from build123d import *

# Parameters (mm, degrees)
ESQUISSE1_R               = 7
ESQUISSE1_R_2             = 6
BOSS_EXTRU_1_DEPTH        = 2.5
BOSS_EXTRU_1_DEPTH_BACK   = 2.5
ESQUISSE1_R_3             = 10.5
ESQUISSE1_R_4             = 9.5
BOSS_EXTRU_1_2_DEPTH      = 2.5
BOSS_EXTRU_1_2_DEPTH_BACK = 2.5
ESQUISSE1_3_R             = 9.5
ESQUISSE1_3_R_2           = 7
BOSS_EXTRU_2_DEPTH        = 2
BOSS_EXTRU_2_DEPTH_BACK   = 2


with BuildPart() as part:
    # Esquisse1 → Boss.-Extru.1 (new body, two sides)
    with BuildSketch(Plane(origin=(0, 0, 0), x_dir=(1, 0, 0), z_dir=(0, 1, 0))) as boss_extru_1_sk:
        Circle(ESQUISSE1_R)
        Circle(ESQUISSE1_R_2, mode=Mode.SUBTRACT)
    extrude(amount=BOSS_EXTRU_1_DEPTH)
    extrude(boss_extru_1_sk.sketch, amount=-BOSS_EXTRU_1_DEPTH_BACK)



with BuildPart() as body_2:
    # Esquisse1 → Boss.-Extru.1 2 (new body, two sides)
    with BuildSketch(Plane(origin=(0, 0, 0), x_dir=(1, 0, 0), z_dir=(0, 1, 0))) as boss_extru_1_2_sk:
        Circle(ESQUISSE1_R_3)
        Circle(ESQUISSE1_R_4, mode=Mode.SUBTRACT)
    extrude(amount=BOSS_EXTRU_1_2_DEPTH)
    extrude(boss_extru_1_2_sk.sketch, amount=-BOSS_EXTRU_1_2_DEPTH_BACK)


with BuildPart() as part_1:
    add(part.part)

    add(body_2.part)  # Boss.-Extru.2 merges body 2
    # Esquisse1_3 → Boss.-Extru.2 (add, two sides)
    with BuildSketch(Plane(origin=(0, 0, 0), x_dir=(1, 0, 0), z_dir=(0, 1, 0))) as boss_extru_2_sk:
        Circle(ESQUISSE1_3_R)
        Circle(ESQUISSE1_3_R_2, mode=Mode.SUBTRACT)
    extrude(amount=BOSS_EXTRU_2_DEPTH)
    extrude(boss_extru_2_sk.sketch, amount=-BOSS_EXTRU_2_DEPTH_BACK)


solid = part_1.part
Part model, mm, in its own coordinate system. A direction names the side the tool comes from. Coordinates: 2 decimals unless noted, no trailing zeros. Order: outer loops, then holes, each group sorted by start corner. A loop starts at its lowest first (then second) coordinate and runs counter-clockwise, first axis right, second up. Notation, with made-up numbers: (18.25, 57) - (31.25, 57) arc R11 cw to (31.25, 75) - close; hole circle Ø2 at (80.5, 62.25). An arc over 180 degrees is marked (long way). Use CSV: the item, a comma, the result in double quotes.
Item 1: Saw through at D-D on y = 1.2. Give the cut face in (x, z), and give its area (3 significant figures).
Solved:
outline,"circle Ø21 at (0, 0); hole circle Ø12 at (0, 0)"
area,"233 mm²"
Item 2: Saw through at A-A on x = 0. Give the cut face in (y, z).
Solved:
outline,"(-2.5, -10.5) - (2.5, -10.5) - (2.5, -9.5) - (2, -9.5) - (2, -7) - (2.5, -7) - (2.5, -6) - (-2.5, -6) - (-2.5, -7) - (-2, -7) - (-2, -9.5) - (-2.5, -9.5) - close; (-2.5, 6) - (2.5, 6) - (2.5, 7) - (2, 7) - (2, 9.5) - (2.5, 9.5) - (2.5, 10.5) - (-2.5, 10.5) - (-2.5, 9.5) - (-2, 9.5) - (-2, 7) - (-2.5, 7) - close"
Item 3: Saw through at B-B on z = 0. Give the cut face in (x, y).
Solved:
outline,"(-10.5, -2.5) - (-9.5, -2.5) - (-9.5, -2) - (-7, -2) - (-7, -2.5) - (-6, -2.5) - (-6, 2.5) - (-7, 2.5) - (-7, 2) - (-9.5, 2) - (-9.5, 2.5) - (-10.5, 2.5) - close; (6, -2.5) - (7, -2.5) - (7, -2) - (9.5, -2) - (9.5, -2.5) - (10.5, -2.5) - (10.5, 2.5) - (9.5, 2.5) - (9.5, 2) - (7, 2) - (7, 2.5) - (6, 2.5) - close"
Item 4: Mould opens along X. For faces 1 (the face through (4.38, -2.25, 8.43)), 2 (the face through (10, 0, -3.2)), 3 (the face through (-5, 2.5, 9)) say: +X half, -X half, draft (parallel to the pull), parting line (faces both ways), or undercut.
Solved:
face 1,"undercut"
face 2,"parting line"
face 3,"draft"
Item 5: 3-axis set-ups, long thin cutter, end or side, ignore diameter. For faces 4 (the face through (4.38, 2.25, 8.43)), 5 (the face through (-4, -2, 6)), 6 (the face through (-6, 0, 0)): which of +Z, -Z, +X, -X, +Y, -Y reach the whole face in a straight line?
Solved:
face 4,"+Y"
face 5,"-Y"
face 6,"+Y, -Y"
Item 6: Drop a flat-ended pin along its axis: P1, Ø1.5, axis at x = 2.5, y = 0, coming from the -Z side. Give the stop position or say it passes through.
Solved:
P1,"stops at z = -10.35"
Item 7: Probe probe 1 along X at (y, z) = (2.2, 0); probe 2 along X at (y, z) = (-0.25, 0). List the from-to ranges inside material, lowest first.
Solved:
probe 1,"x = -10.5 to -9.5, -7 to -6, 6 to 7, 9.5 to 10.5"
probe 2,"x = -10.5 to -6, 6 to 10.5"
Item 8: Saw through at C-C on x = 6.5. Give the cut face in (y, z).
Solved:
outline,"(-2.5, -8.25) - (2.5, -8.25) - (2.5, -6.93) - (2, -6.93) - (2, -2.6) - (2.5, -2.6) - (2.5, 2.6) - (2, 2.6) - (2, 6.93) - (2.5, 6.93) - (2.5, 8.25) - (-2.5, 8.25) - (-2.5, 6.93) - (-2, 6.93) - (-2, 2.6) - (-2.5, 2.6) - (-2.5, -2.6) - (-2, -2.6) - (-2, -6.93) - (-2.5, -6.93) - close"
